Part model, mm, in its own coordinate system. A direction names the side the tool comes from. Coordinates: 2 decimals unless noted, no trailing zeros. Order: outer loops, then holes, each group sorted by start corner. A loop starts at its lowest first (then second) coordinate and runs counter-clockwise, first axis right, second up.
1) Pin check, flat tips, straight feed: pin 1 Ø0.6 at (x, z) = (43, 1) entering from -Y; pin 2 Ø1.2 at (x, z) = (-45, 3) entering from -Y; pin 3 Ø1.2 at (y, z) = (-25.5, 2) entering from +X. Stop position of each tip, or through.
2) Tool access for faces 1 (the flat face through (42.5, -25, 2)), 2 (the cylindrical face through (40.3, -20.4, 2.3)), 3 (the flat face through (39.5, -24, 2)), 4 (the flat face through (-44, 36.5, 3)): list every direction of +Z, -Z, +X, -X, +Y, -Y with a clear straight run to the whole face (end or side of a thin tool).
3) Cut at A-A (y = 24). List the corners of the cut face in (x, z).
4) Wall check: L1, parallel to X at y = -3.5, z = 1.95; L2, parallel to Y at x = 1, z = 3.5; L3, parallel to X at y = 14, z = 4.15. Give the ranges that are in metal, low to high.
5) Mould opens along X. For faces 5 (the flat face through (46.5, 9, 2)), 6 (the flat face through (45, 39.5, 2)), 7 (the cylindrical face through (40.3, 37.4, 2.3)) say: +X half, -X half, draft (parallel to the pull), parting line (faces both ways), or undercut.
6) Cut at C-C (x = 25.5). List the corners of the cut face in (y, z), and give its area (3 significant figures).
```python
from build123d import *

# Parameters (mm, degrees)
PAD001_DEPTH   = 4.6
SKETCH001003_W = 3
SKETCH001003_H = 56
POCKET_DEPTH   = 2.6
FILLET_R       = 1.5
FILLET001_R    = 2.9


with BuildPart() as part:
    # Sketch001002 → Pad001 (new body)
    with BuildSketch(Plane.XY):
        Polygon((-46.5, 39.5), (-42.5, 39.5), (-42.5, 43.5), (42.5, 43.5), (42.5, 39.5), (46.5, 39.5), (46.5, -22.5), (42.5, -22.5), (42.5, -26.5), (39.5, -26.5), (39.5, -19.5), (43.5, -19.5), (43.5, 36.5), (39.5, 36.5), (39.5, 40.5), (-39.5, 40.5), (-39.5, 36.5), (-43.5, 36.5), (-43.5, -19.5), (-39.5, -19.5), (-39.5, -26.5), (-42.5, -26.5), (-42.5, -22.5), (-46.5, -22.5), align=None)
    extrude(amount=PAD001_DEPTH)

    # Sketch001003 → Pocket (cut)
    with BuildSketch(Plane.XY.offset(4.6)):
        with Locations((-45, 8.5)):
            Rectangle(SKETCH001003_W, SKETCH001003_H)
    extrude(amount=-POCKET_DEPTH, mode=Mode.SUBTRACT)

    # Fillet
    fillet_edges = [part.edges().sort_by_distance(p)[0] for p in [
        (42.5, -22.5, 2.3),
        (42.5, 39.5, 2.3),
        (-42.5, 39.5, 2.3),
        (-42.5, -22.5, 2.3),
    ]]
    fillet(fillet_edges, radius=FILLET_R)

    # Fillet001
    fillet001_edges = [part.edges().sort_by_distance(p)[0] for p in [
        (39.5, 36.5, 2.3),
        (39.5, -19.5, 2.3),
        (-39.5, 36.5, 2.3),
        (-39.5, -19.5, 2.3),
    ]]
    fillet(fillet001_edges, radius=FILLET001_R)


solid = part.part
```
Geometry check:
1. pin 1: stops at y = -23.25
1. pin 2: stops at y = -22.5
1. pin 3: stops at x = 42.5
2. face 1: +Z, -Z, +X, -Y
2. face 2: +Z, -Z
2. face 3: +Z, -Z, -Y
2. face 4: +Z
3. outline: (-46.5, 0) - (-43.5, 0) - (-43.5, 2) - (-46.5, 2) - close; (43.5, 0) - (46.5, 0) - (46.5, 4.6) - (43.5, 4.6) - close
4. L1: x = -46.5 to -43.5, 43.5 to 46.5
4. L2: y = 40.5 to 43.5
4. L3: x = 43.5 to 46.5
5. face 5: +X half
5. face 6: draft
5. face 7: undercut
6. outline: (40.5, 0) - (43.5, 0) - (43.5, 4.6) - (40.5, 4.6) - close
6. area: 13.8 mm2
